from build123d import *

# Parameters (mm, degrees)
SKETCH1_W             = 69.85
SKETCH1_H             = 50.8
BASE_DEPTH            = 5.999988
SKETCH6_W             = 12.7
SKETCH6_H             = 5.999988
BOSS_EXTRUDE1_DEPTH   = 5.999988
SKETCH7_W             = 25.4
SKETCH7_H             = 41.275
CUT_EXTRUDE1_DEPTH    = 48.346749914
F_8_CLEARANCE_HOLE1_D = 4.3053
SKETCH8_W             = 25.4
SKETCH8_H             = 41.275
CUT_EXTRUDE2_DEPTH    = 48.346749914
FILLET1_R             = 5.08


with BuildPart() as part:
    # Sketch1 → Base (new body)
    with BuildSketch(Plane.XY):
        Rectangle(SKETCH1_W, SKETCH1_H)
    extrude(amount=BASE_DEPTH)

    # Sketch6 → Boss-Extrude1 (add)
    with BuildSketch(Plane.XY.offset(5.999988)):
        with Locations((0, 28.399994)):
            Rectangle(SKETCH6_W, SKETCH6_H)
        with Locations((28.575, -28.399994)):
            Rectangle(SKETCH6_W, SKETCH6_H)
        with Locations((-28.575, -28.399994)):
            Rectangle(SKETCH6_W, SKETCH6_H)
    extrude(amount=-BOSS_EXTRUDE1_DEPTH)

    # Sketch7 → Cut-Extrude1 (cut, through all)
    with BuildSketch(Plane.XY.offset(5.999988)):
        with Locations((-22.225, 4.7625)):
            Rectangle(SKETCH7_W, SKETCH7_H)
    extrude(amount=-CUT_EXTRUDE1_DEPTH, mode=Mode.SUBTRACT)

    # #8 Clearance Hole1 (through all)
    with Locations(Plane(origin=(0, 0, 0), x_dir=(-1, 0, 0), z_dir=(0, 0, -1))):
        with Locations((0, -20.6375), (0, -7.9375), (0, 4.7625)):
            Hole(F_8_CLEARANCE_HOLE1_D / 2)

    # Sketch8 → Cut-Extrude2 (cut, through all)
    with BuildSketch(Plane.XY.offset(5.999988)):
        with Locations((22.225, 4.7625)):
            Rectangle(SKETCH8_W, SKETCH8_H)
    extrude(amount=-CUT_EXTRUDE2_DEPTH, mode=Mode.SUBTRACT)

    # Fillet1
    fillet1_edges = [part.edges().sort_by_distance(p)[0] for p in [
        (34.925, -15.875, 2.999994),
        (9.525, -15.875, 2.999994),
        (-9.525, -15.875, 2.999994),
        (-34.925, -15.875, 2.999994),
    ]]
    fillet(fillet1_edges, radius=FILLET1_R)


solid = part.part
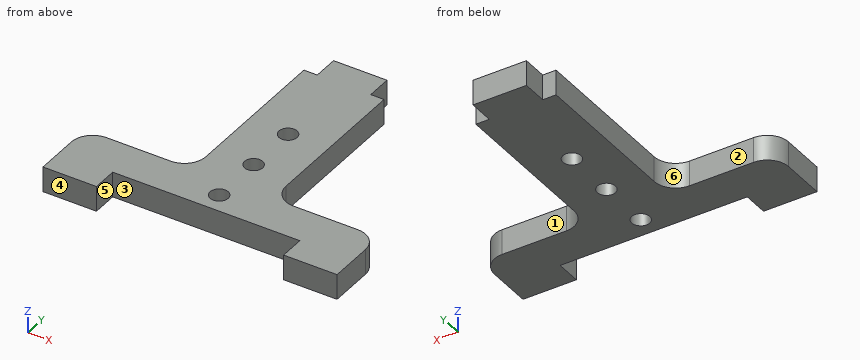
Geometry: final body of the model. Coordinates: model frame, mm. Face numbers are marked on the shaded views. A direction names the side the tool comes from. Round coordinates to 2 decimals unless told otherwise and drop trailing zeros. Order: outer loops, then holes, each group sorted by start corner. A loop starts at its lowest first (then second) coordinate and runs counter-clockwise, first axis right, second up.
Q1. Section A-A, the plane y = -27. Output: boundary loops of the cut face in (x, z) (3 decimals).
Result sheet:
outline: (-34.925, 0) - (-22.225, 0) - (-22.225, 6) - (-34.925, 6) - close; (22.225, 0) - (34.925, 0) - (34.925, 6) - (22.225, 6) - close
Q2. Section D-D, the plane x = -15.5. Output: boundary loops of the cut face in (y, z) (3 decimals), and give its area (4 significant figures).
Result sheet:
outline: (-25.4, 0) - (-15.875, 0) - (-15.875, 6) - (-25.4, 6) - close
area: 57.15 mm2
Q3. Section C-C, the plane z = 0.95. Give the number of separate pieces and of enclosed holes in the cut face, and give its area (3 significant figures).
Result sheet:
separate pieces: 1
enclosed holes: 3
area: 1,640 mm2
Q4. Mould query, pull axis X, two halves, no side actions, for the marked faces 4, 5 and 6. Classes: released by +X, released by -X, zero draft, split by the parting line, or undercut.
Result sheet:
face 4: zero draft
face 5: undercut
face 6: released by -X
Q5. Pin query (flat end, axial travel): pin 1 (3 mm diameter, centred on y = 12.5, z = 3.5, fed in from +X) (3 decimals); pin 2 (2.5 mm diameter, centred on x = -8, z = 3.5, fed in from +Y); pin 3 (1.5 mm diameter, centred on x = 20, z = 3.5, fed in from +Y) (3 decimals). Return the tip coordinate at first contact, or that it passes through.
Result sheet:
pin 1: stops at x = 9.525
pin 2: stops at y = 25.4
pin 3: stops at y = -15.875
Q6. Section B-B, the plane x = 0. Output: boundary loops of the cut face in (y, z), and give its area (3 significant figures).
Result sheet:
outline: (-25.4, 0) - (-22.79, 0) - (-22.79, 6) - (-25.4, 6) - close; (-18.48, 0) - (-10.09, 0) - (-10.09, 6) - (-18.48, 6) - close; (-5.78, 0) - (2.61, 0) - (2.61, 6) - (-5.78, 6) - close; (6.92, 0) - (31.4, 0) - (31.4, 6) - (6.92, 6) - close
area: 263 mm2
Q7. Access query for the marked faces 1, 2 and 3. Directions: +Z, -Z, +X, -X, +Y, -Y. A direction counts if a zero-diameter tool reaches every point of the face in a straight line with its end or side. Return the directions, or none.
Result sheet:
face 1: +Z, -Z, +X, +Y
face 2: +Z, -Z, -X, +Y
face 3: +Z, -Z, -Y
Q8. Material intervals for probe 1 along Y at (x, z) = (0, 2); probe 2 along X at (y, z) = (5, 3.9) (1 decimal); probe 3 along X at (y, z) = (-11, 3), sorted ascending.
Result sheet:
probe 1: y = -25.4 to -22.79, -18.48 to -10.09, -5.78 to 2.61, 6.92 to 31.4
probe 2: x = -9.5 to -2.1, 2.1 to 9.5
probe 3: x = -9.53 to 9.53
